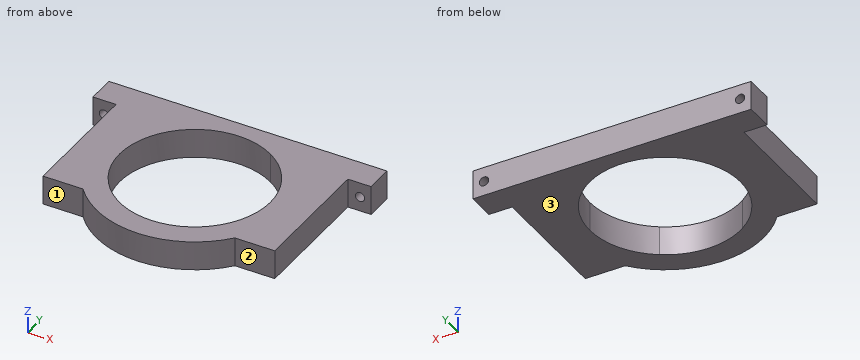
```python
from build123d import *

# Parameters (mm, degrees)
F1_DEPTH = 12.6
F2_R     = 2
F3_DEPTH = 82.4149229208


# Not quite as in the source:
# - a feature names something its author has since deleted; it is built from what else it names


with BuildPart() as f1:
    # F0 (on Top) → F1 (new body)
    with BuildSketch(Plane.XY):
        with BuildLine():
            Line((4.3273164821, 32.1861776987), (-41.0737535205, 32.1861776987))
            Line((-41.0737535205, 32.1861776987), (-41.0737535205, 20.1861776987))
            Line((-41.0737535205, 20.1861776987), (-31.0737535205, 20.1861776987))
            Line((-31.0737535205, 20.1861776987), (-13.1215757112, 20.1861776987))
            ThreePointArc((-13.1215757112, 20.1861776987), (-5.1565247985, 27.2903947567), (4.3273164821, 32.1861776987))
        make_face()
        with BuildLine():
            Line((33.525176477, 32.1861776987), (4.3273164821, 32.1861776987))
            ThreePointArc((4.3273164821, 32.1861776987), (-5.1565247985, 27.2903947567), (-13.1215757112, 20.1861776987))
            Line((-13.1215757112, 20.1861776987), (2.2810397469, 20.1861776987))
            ThreePointArc((2.2810397469, 20.1861776987), (18.9262464795, 24.7722547779), (35.5714532121, 20.1861776987))
            Line((35.5714532121, 20.1861776987), (50.9740686703, 20.1861776987))
            ThreePointArc((50.9740686703, 20.1861776987), (43.0090177575, 27.2903947567), (33.525176477, 32.1861776987))
        make_face()
        with BuildLine():
            Line((78.9262464795, 32.1861776987), (33.525176477, 32.1861776987))
            ThreePointArc((33.525176477, 32.1861776987), (43.0090177575, 27.2903947567), (50.9740686703, 20.1861776987))
            Line((50.9740686703, 20.1861776987), (68.9262464795, 20.1861776987))
            Line((68.9262464795, 20.1861776987), (78.9262464795, 20.1861776987))
            Line((78.9262464795, 20.1861776987), (78.9262464795, 32.1861776987))
        make_face()
        with BuildLine():
            Line((68.9262464795, 20.1861776987), (50.9740686703, 20.1861776987))
            ThreePointArc((50.9740686703, 20.1861776987), (58.7275180868, 7.1755691223), (61.4262464795, -7.7277452221))
            ThreePointArc((61.4262464795, -7.7277452221), (58.9146555301, -22.121394572), (51.6767339333, -34.8138223013))
            Line((51.6767339333, -34.8138223013), (68.9262464795, -34.8138223013))
            Line((68.9262464795, -34.8138223013), (68.9262464795, 20.1861776987))
        make_face()
        with BuildLine():
            ThreePointArc((-13.8242409743, -34.8138223013), (-23.5702855343, -7.1848209158), (-13.1215757112, 20.1861776987))
            Line((-13.1215757112, 20.1861776987), (-31.0737535205, 20.1861776987))
            Line((-31.0737535205, 20.1861776987), (-31.0737535205, -34.8138223013))
            Line((-31.0737535205, -34.8138223013), (-19.9806198337, -34.8138223013))
            Line((-19.9806198337, -34.8138223013), (-13.8242409743, -34.8138223013))
        make_face()
        with BuildLine():
            Line((2.2810397469, 20.1861776987), (-13.1215757112, 20.1861776987))
            ThreePointArc((-13.1215757112, 20.1861776987), (-23.5702855343, -7.1848209158), (-13.8242409743, -34.8138223013))
            Line((-13.8242409743, -34.8138223013), (0.9653325701, -34.8138223013))
            ThreePointArc((0.9653325701, -34.8138223013), (-13.5644582908, -6.9505042503), (2.2810397469, 20.1861776987))
        make_face()
        with BuildLine():
            ThreePointArc((61.4262464795, -7.7277452221), (58.7275180868, 7.1755691223), (50.9740686703, 20.1861776987))
            Line((50.9740686703, 20.1861776987), (35.5714532121, 20.1861776987))
            ThreePointArc((35.5714532121, 20.1861776987), (47.1859281728, 8.3234351269), (51.4262464795, -7.7277452221))
            ThreePointArc((51.4262464795, -7.7277452221), (47.5617113968, -23.0985015136), (36.8871603889, -34.8138223013))
            Line((36.8871603889, -34.8138223013), (51.6767339333, -34.8138223013))
            ThreePointArc((51.6767339333, -34.8138223013), (58.9146555301, -22.121394572), (61.4262464795, -7.7277452221))
        make_face()
        with BuildLine():
            Line((0.9653325701, -34.8138223013), (-13.8242409743, -34.8138223013))
            ThreePointArc((-13.8242409743, -34.8138223013), (18.9262464795, -50.2277452221), (51.6767339333, -34.8138223013))
            Line((51.6767339333, -34.8138223013), (36.8871603889, -34.8138223013))
            ThreePointArc((36.8871603889, -34.8138223013), (18.9262464795, -40.2277452221), (0.9653325701, -34.8138223013))
        make_face()
    extrude(amount=F1_DEPTH)

    # F2 (on face) → F3 (cut, through all)
    with BuildSketch(Plane(origin=(0, 32.1861776987, 0), x_dir=(-1, 0, 0), z_dir=(0, 1, 0))):
        with Locations((-74.1762464795, 6.3)):
            Circle(F2_R)
        with Locations((36.3237535205, 6.3)):
            Circle(F2_R)
    extrude(amount=-F3_DEPTH, mode=Mode.SUBTRACT)


solid = f1.part
```
Can you work these out from the model? Positions are in its coordinate system, mm. Face numbers are marked on the shaded views. A direction names the side the tool comes from. Coordinates: 2 decimals unless noted, no trailing zeros. Write each loop counter-clockwise with the first axis right and the second up, starting at its lowest first coordinate (ties: lowest second). Pieces come first, ordered by that corner, then holes. Notation, with made-up numbers: M -31.5,-39 L -20.5,-39 A18 ccw -20.5,-18 Z; hole C 0.5,-28 d5. An arc over 180 degrees is marked long. Write item = value, one per line. Start each with the question number.
Q1. On a 3-axis mill with a long thin cutter (end or side, diameter ignored), from which of +Z, -Z, +X, -X, +Y, -Y can I reach the whole of each face in a straight line? I mean the marked faces 1, 2 and 3. Say none if no direction works.
Q2. If I drill on L1, parallel to Y at x = 18.5, z = 1; L2, parallel to X at y = 6.5, z = 5.5; L3, parallel to Y at x = -23.5, z = 0.75, over which ranges is the centre line in solid material (lowest first)? Write a range as [from, to].
Q3. I'm going to push flat-ended pins straight in: pin 1 (1 mm diameter, centred on x = 30.5, z = 7, fed in from -Y); pin 2 (1.5 mm diameter, centred on y = -30.5, z = 7.5, fed in from +X); pin 3 (5 mm diameter, centred on x = 75, z = 7, fed in from -Y). Where does each tip first touch, or does it pass through?
Q4. If we section it at A-A, the plane z = 6.3: Write out the boundary of the cut face in (x, y), then the cut area to 3 significant figures.
Q5. If we section it at C-C, the plane x = 46.5: Write out the boundary of the cut face in (y, z).
Q6. If we section it at B-B, the plane y = 13.5: Write out the boundary of the cut face in (x, z), then the cut area to 3 significant figures.
Check sheet entries:
q1.face_1 = +Z, -Z, -X, -Y
q1.face_2 = +Z, -Z, +X, -Y
q1.face_3 = -Z, +X, -X, +Y, -Y
q2.L1 = [-50.23, -40.22], [24.77, 32.19]
q2.L2 = [-31.07, -10.29], [48.15, 68.93]
q2.L3 = [-34.81, 32.19]
q3.pin_1 = -48.76
q3.pin_2 = 68.93
q3.pin_3 = 20.19
q4.outline = M -41.07,20.19 L -38.32,20.19 L -38.32,32.19 L -41.07,32.19 Z; M -34.32,20.19 L -31.07,20.19 L -31.07,-34.81 L -13.82,-34.81 A42.5 ccw 51.68,-34.81 L 68.93,-34.81 L 68.93,20.19 L 72.18,20.19 L 72.18,32.19 L -34.32,32.19 Z; M 76.18,20.19 L 78.93,20.19 L 78.93,32.19 L 76.18,32.19 Z; hole C 18.93,-7.73 d65
q4.area = 4,230 mm²
q5.outline = M -40.07,0 L -24.93,0 L -24.93,12.6 L -40.07,12.6 Z; M 9.48,0 L 32.19,0 L 32.19,12.6 L 9.48,12.6 Z
q6.outline = M -31.07,0 L -5.68,0 L -5.68,12.6 L -31.07,12.6 Z; M 43.54,0 L 68.93,0 L 68.93,12.6 L 43.54,12.6 Z
q6.area = 640 mm²
